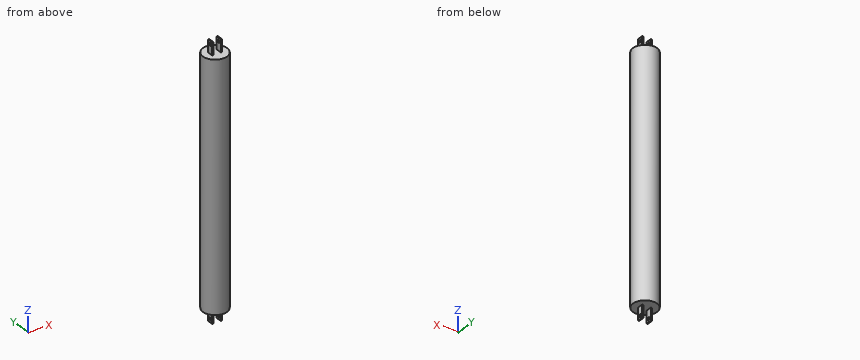
from build123d import *

# Parameters (mm, degrees)
SKETCH1_R           = 20
BOSS_EXTRUDE1_DEPTH = 200
SKETCH2_W           = 1.819488692
SKETCH2_H           = 20.46
BOSS_EXTRUDE2_DEPTH = 5
SKETCH3_R           = 2.5
CUT_EXTRUDE1_DEPTH  = 9


with BuildPart() as part:
    # Sketch1 → Boss-Extrude1 (new, symmetric)
    with BuildSketch(Plane.XY):
        Circle(SKETCH1_R)
    extrude(amount=BOSS_EXTRUDE1_DEPTH, both=True)

    # Sketch2 → Boss-Extrude2 (add, symmetric)
    with BuildSketch(Plane(origin=(0, 0, 0), x_dir=(1, 0, 0), z_dir=(0, 1, 0))):
        with Locations((7.090255654, -210.23)):
            Rectangle(SKETCH2_W, SKETCH2_H)
        with Locations((-7.090255654, -210.23)):
            Rectangle(SKETCH2_W, SKETCH2_H)
        with Locations((7.090255654, 210.23)):
            Rectangle(SKETCH2_W, SKETCH2_H)
        with Locations((-7.090255654, 210.23)):
            Rectangle(SKETCH2_W, SKETCH2_H)
    extrude(amount=BOSS_EXTRUDE2_DEPTH, both=True)

    # Sketch3 → Cut-Extrude1 (cut, symmetric)
    with BuildSketch(Plane(origin=(0, 0, 0), x_dir=(0, 0, -1), z_dir=(1, 0, 0))):
        with Locations((-215, 0)):
            Circle(SKETCH3_R)
        with Locations(Location((215, 0, 0), (0, 0, 180))):
            Circle(SKETCH3_R)
    extrude(amount=CUT_EXTRUDE1_DEPTH, both=True, mode=Mode.SUBTRACT)


solid = part.part
The model under review builds one solid part; all positions refer to its coordinate system, in mm. Coordinates: 2 decimals unless noted, no trailing zeros. Write each loop counter-clockwise with the first axis right and the second up, starting at its lowest first coordinate (ties: lowest second). Pieces come first, ordered by that corner, then holes. Notation, with made-up numbers: (78, 78) - (104, 78) arc R16 ccw to (104, 97) - close; hole circle Ø1 at (-11, -33.75). An arc over 180 degrees is marked (long way). Answer as CSV lines item,"result".
(1) Clearance check with flat-ended pins moving along their axes: pin 1 Ø5 at (x, z) = (13.5, -14.5) entering from +Y; pin 2 Ø5 at (y, z) = (1, 205.5) entering from +X; pin 3 Ø8 at (y, z) = (-2, -205.5) entering from -X; pin 4 Ø4 at (y, z) = (0, -215) entering from -X. State where each tip first meets the part, or that it passes through.
Data:
pin 1,"stops at y = 16.7"
pin 2,"stops at x = 8"
pin 3,"stops at x = -8"
pin 4,"passes through"
(2) We need section C-C (y = -14.5). Give the boundary of the cut face in (x, z), plus the area to 3 significant figures.
Data:
outline,"(-13.77, -200) - (13.77, -200) - (13.77, 200) - (-13.77, 200) - close"
area,"11,000 mm2"
(3) We need section B-B (z = -54.5). Give the boundary of the cut face in (x, y).
Data:
outline,"circle Ø40 at (0, 0)"
(4) For line 1 along X through (y, z) = (0.5, 201); line 2 along Y through (x, z) = (-7.2, 215); line 3 along Z through (x, y) = (9.5, 10), list the stretches that pass through material, from the lowest coordinate up. Write a range as [from, to].
Data:
line 1,"x = [-8, -6.18], [6.18, 8]"
line 2,"y = [-5, -2.5], [2.5, 5]"
line 3,"z = [-200, 200]"
(5) We need section A-A (x = 0). Give the boundary of the cut face in (y, z).
Data:
outline,"(-20, -200) - (20, -200) - (20, 200) - (-20, 200) - close"
